Part model, mm, in its own coordinate system. A direction names the side the tool comes from. Round coordinates to 2 decimals unless told otherwise and drop trailing zeros. Loops run counter-clockwise (first coordinate to the right, second up) from the corner with the lowest first, then second, coordinate; pieces in that order, holes last. Notation, with made-up numbers: (-3.75, 20) - (4.25, 20) arc R18 ccw to (4.25, 53) - close; hole circle Ø1 at (42.5, 11). An arc over 180 degrees is marked (long way). Put each result on its own line as item: value.
from build123d import *

# Parameters (mm, degrees)
SKETCH1_R           = 1.9
BOSS_EXTRUDE1_DEPTH = 30
SKETCH3_R           = 6.607376419
SKETCH3_R_2         = 1.965008769
BOSS_EXTRUDE2_DEPTH = 0.2


with BuildPart() as part:
    # Sketch1 → Boss-Extrude1 (new body)
    with BuildSketch(Plane(origin=(0, 0, 0), x_dir=(1, 0, 0), z_dir=(0, 1, 0))):
        Polygon((1.964165255, -3.532051555), (4.040929001, -0.065008769), (2.076763746, 3.467042785), (-1.964165255, 3.532051555), (-4.040929001, 0.065008769), (-2.076763746, -3.467042785), align=None)
        with Locations((0, 0.065008769)):
            Circle(SKETCH1_R, mode=Mode.SUBTRACT)
    extrude(amount=BOSS_EXTRUDE1_DEPTH)

    # Sketch3 → Boss-Extrude2 (add)
    with BuildSketch(Plane(origin=(0, 0, 0), x_dir=(-1, 0, 0), z_dir=(0, -1, 0))):
        Circle(SKETCH3_R)
        Circle(SKETCH3_R_2, mode=Mode.SUBTRACT)
    extrude(amount=-BOSS_EXTRUDE2_DEPTH)


solid = part.part
1. Band-saw the part on D-D (x = 1.5). List the corners of the cut face in (y, z), plus the area to 3 significant figures.
A:
outline: (0, -6.43) - (0.2, -6.43) - (0.2, -3.48) - (30, -3.48) - (30, -1.23) - (0, -1.23) - close; (0, 1.1) - (30, 1.1) - (30, 3.52) - (0.2, 3.52) - (0.2, 6.43) - (0, 6.43) - close
area: 141 mm²
2. Band-saw the part on C-C (z = -3). List the corners of the cut face in (x, y).
A:
outline: (-5.89, 0) - (5.89, 0) - (5.89, 0.2) - (2.34, 0.2) - (2.34, 30) - (-2.28, 30) - (-2.28, 0.2) - (-5.89, 0.2) - close
3. Band-saw the part on B-B (x = 0). List the corners of the cut face in (y, z) (3 decimals), plus the area to 3 significant figures.
A:
outline: (0, -6.607) - (0.2, -6.607) - (0.2, -3.5) - (30, -3.5) - (30, -1.965) - (0, -1.965) - close; (0, 1.835) - (30, 1.835) - (30, 3.5) - (0.2, 3.5) - (0.2, 6.607) - (0, 6.607) - close
area: 97.3 mm²
4. Probe line 1 along X through (y, z) = (26, -1); line 2 along Z through (x, y) = (0, 21.25) (3 decimals); line 3 along Y through (x, z) = (-0.25, -4.25). List the from-to ranges inside material, lowest first. Write a range as [from, to].
A:
line 1: x = [-3.48, -1.65], [1.65, 3.45]
line 2: z = [-3.5, -1.965], [1.835, 3.5]
line 3: y = [0, 0.2]
5. Tool access for faces 5 (the flat face through (3, 14.9, 1.8)), 6 (the flat face through (-3, 0.2, 3)), 7 (the flat face through (-3, 14.9, -1.8)): list every direction of +Z, -Z, +X, -X, +Y, -Y with a clear straight run to the whole face (end or side of a thin tool).
A:
face 5: +Z, +X, +Y
face 6: +Y
face 7: -Z, -X, +Y
6. Two-plate mould, pull along X, no slides. Class faces 1 (the flat face through (-3.07, 14.89, 1.68)), 2 (the flat face through (-1, 0, -2)), 3 (the cylindrical face through (-0.41, 14.79, 1.79)), 4 (the flat face through (3.07, 14.89, -1.68)): pulls with the +X half, pulls with the -X half, needs draft (parallel to the pull), parting line crosses it, or undercut.
A:
face 1: pulls with the -X half
face 2: needs draft
face 3: undercut
face 4: pulls with the +X half
7. Band-saw the part on A-A (y = 25.75). List the corners of the cut face in (x, z) (3 decimals), plus the area to 3 significant figures.
A:
outline: (-4.041, -0.065) - (-1.964, -3.532) - (2.077, -3.467) - (4.041, 0.065) - (1.964, 3.532) - (-2.077, 3.467) - close; hole circle Ø3.8 at (0, -0.065)
area: 31.1 mm²
8. Pin check, flat tips, straight feed: P1, Ø3, axis at x = 0, z = -0.07, coming from the +Y side; P2, Ø1.5, axis at y = 7.5, z = 0.5, coming from the -X side; P3, Ø3, axis at y = 16.5, z = 0, coming from the +X side; P4, Ø2, axis at x = 5, z = -1, coming from the +Y side. Stop position of each tip, or through.
A:
P1: passes through
P2: stops at x = -4.04
P3: stops at x = 4.04
P4: stops at y = 0.2
